Geometry: final body of the model. Coordinates: model frame, mm. Face numbers are marked on the shaded views. A direction names the side the tool comes from. Round coordinates to 2 decimals unless told otherwise and drop trailing zeros. Order: outer loops, then holes, each group sorted by start corner. A loop starts at its lowest first (then second) coordinate and runs counter-clockwise, first axis right, second up. Notation, with made-up numbers: M -11.5,25.5 L 34.5,25.5 A9 cw 34.5,30.5 Z; hole C 55,63 d7. An arc over 180 degrees is marked long. Return JSON: item names as keys, results as strings. Group by question number.
Q1. Cut plane C-C on z = -19. Output: boundary loops of the cut face in (x, y).
Q2. Contact query for flat-ended pins moving along their axis: pin 1 (23 mm diameter, centred on x = 31.5, y = 38, fed in from -Z); pin 2 (1.5 mm diameter, centred on x = -31, z = -38, fed in from -Y); pin 3 (5 mm diameter, centred on x = -1, z = -33.5, fed in from -Y). Output: stop coordinate, or through.
Q3. Cut plane D-D on x = 35.5. Output: boundary loops of the cut face in (y, z), and give its area (3 significant figures).
Q4. Access query for the marked faces 1, 2 and 3. Directions: +Z, -Z, +X, -X, +Y, -Y. A direction counts if a zero-diameter tool reaches every point of the face in a straight line with its end or side. Return the directions, or none.
Q5. Cut plane A-A on x = -50.5. Output: boundary loops of the cut face in (y, z).
Q6. Ray query, probe 1 along Z at (x, y) = (46, 48); probe 2 along Z at (x, y) = (24.5, 81); probe 3 along Y at (x, z) = (-0.5, -10). Return the intervals inside material, ascending.
Q7. Cut plane B-B on y = 20. Output: boundary loops of the cut face in (x, z), and give its area (3 significant figures).
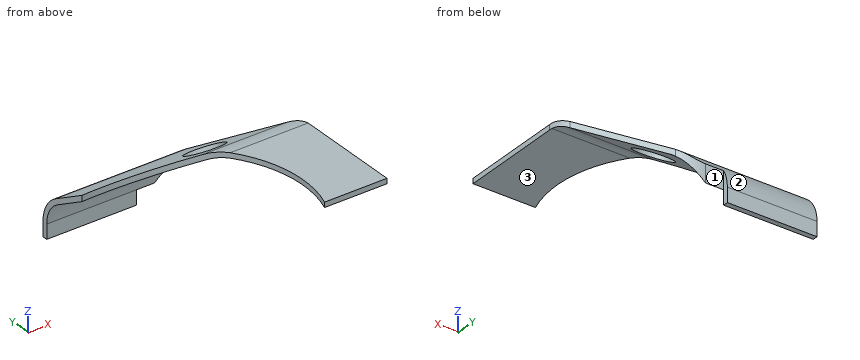
```python
from build123d import *

# Parameters (mm, degrees)
SALIENTE_EXTRUIR1_DEPTH = 58.05
REDONDEO1_R             = 20
REDONDEO2_R             = 20
REDONDEO3_R             = 17
REDONDEO4_R             = 17
CAVIDAD1_START          = -47
CAVIDAD1_DEPTH          = 50
CROQUIS16_R             = 67.5
CORTAR_EXTRUIR11_DEPTH  = 143.339628461
CROQUIS18_R             = 11
CORTAR_EXTRUIR12_DEPTH  = 142.06007654


# Read off the part's stored shape, not the designer's step: Cavidad1
with BuildPart() as part:
    # Croquis1 → Saliente-Extruir1 (new, symmetric)
    with BuildSketch(Plane(origin=(0, 0, 0), x_dir=(0, 0, -1), z_dir=(1, 0, 0))):
        Polygon((0, 0), (0, 67.196152423), (28.732050808, 116.961524227), (47, 116.961524227), (47, 119.961524227), (27, 119.961524227), (-3, 68), (-3, 0), align=None)
    extrude(amount=SALIENTE_EXTRUIR1_DEPTH, both=True)

    # Redondeo1
    redondeo1_edges = [part.edges().sort_by_distance(p)[0] for p in [
        (0, 68, 3),
    ]]
    fillet(redondeo1_edges, radius=REDONDEO1_R)

    # Redondeo2
    redondeo2_edges = [part.edges().sort_by_distance(p)[0] for p in [
        (0, 119.961524227, -27),
    ]]
    fillet(redondeo2_edges, radius=REDONDEO2_R)

    # Redondeo3
    redondeo3_edges = [part.edges().sort_by_distance(p)[0] for p in [
        (0, 116.961524227, -28.732050808),
    ]]
    fillet(redondeo3_edges, radius=REDONDEO3_R)

    # Redondeo4
    redondeo4_edges = [part.edges().sort_by_distance(p)[0] for p in [
        (0, 67.196152423, 0),
    ]]
    fillet(redondeo4_edges, radius=REDONDEO4_R)

    # Cavidad1 outline → Cavidad1 (cut)
    with BuildSketch(Plane.XY.offset(CAVIDAD1_START)):
        with BuildLine():
            Line((58.05, 0), (58.05, 119.961524227))
            Line((58.05, 119.961524227), (-5.55, 119.961524227))
            Line((-5.55, 119.961524227), (-5.55, 116.961524227))
            Line((-5.55, 116.961524227), (5.123846837, 116.961524227))
            ThreePointArc((5.123846837, 116.961524227), (12.308357287, 115.368756607), (18.14660237, 110.888913592))
            Line((18.14660237, 110.888913592), (51.073651347, 71.647984679))
            ThreePointArc((51.073651347, 71.647984679), (54.025670368, 66.534937751), (55.050895814, 60.720595315))
            Line((55.050895814, 60.720595315), (55.050895814, 0))
            Line((55.050895814, 0), (58.05, 0))
        make_face()
    extrude(amount=CAVIDAD1_DEPTH, mode=Mode.SUBTRACT)

    # Croquis16 → Cortar-Extruir11 (cut, through all)
    with BuildSketch(Plane.XY.offset(3)):
        with Locations((-45.071920691, 22.721524227)):
            Circle(CROQUIS16_R)
    extrude(amount=-CORTAR_EXTRUIR11_DEPTH, mode=Mode.SUBTRACT)

    # Croquis18 → Cortar-Extruir12 (cut, through all)
    with BuildSketch(Plane(origin=(0, 18.299038106, 31.694863729), x_dir=(1, 0, 0), z_dir=(0, 0.4999999999999976, 0.86602540378444))):
        with Locations(Location((12.350895814, 79.099876042, 0), (0, 0, 270))):
            Circle(CROQUIS18_R)
    extrude(amount=-CORTAR_EXTRUIR12_DEPTH, mode=Mode.SUBTRACT)


solid = part.part
```
Result sheet:
{
 "1": {"outline": "M -58.05,100.11 L 27.2,100.11 L 22.16,106.11 L -58.05,106.11 Z"},
 "2": {"pin 1": "stops at z = 0", "pin 2": "stops at y = 116.91", "pin 3": "stops at y = 115.19"},
 "3": {"outline": "M 0,0 L 62.64,0 A17 cw 71.14,-2.28 L 90.21,-13.29 L 90.21,-9.82 L 72.64,0.32 A20 ccw 62.64,3 L 0,3 Z", "area": "280 mm²"},
 "4": {"face 1": "+Z, -Z, +X, +Y", "face 2": "+Z, +X, -X, +Y", "face 3": "-Z, +X, -X, -Y"},
 "5": {"outline": "M 90,-13.17 L 108.46,-23.82 A17 cw 116.96,-38.55 L 116.96,-47 L 119.96,-47 L 119.96,-38.55 A20 ccw 109.96,-21.23 L 90,-9.7 Z"},
 "6": {"probe 1": "z = 0 to 3", "probe 2": "z = -7.97 to -4.51", "probe 3": "y = 84.52 to 90.52"},
 "7": {"outline": "M 22.37,0 L 55.05,0 L 55.05,3 L 22.37,3 Z", "area": "98.0 mm²"}
}
